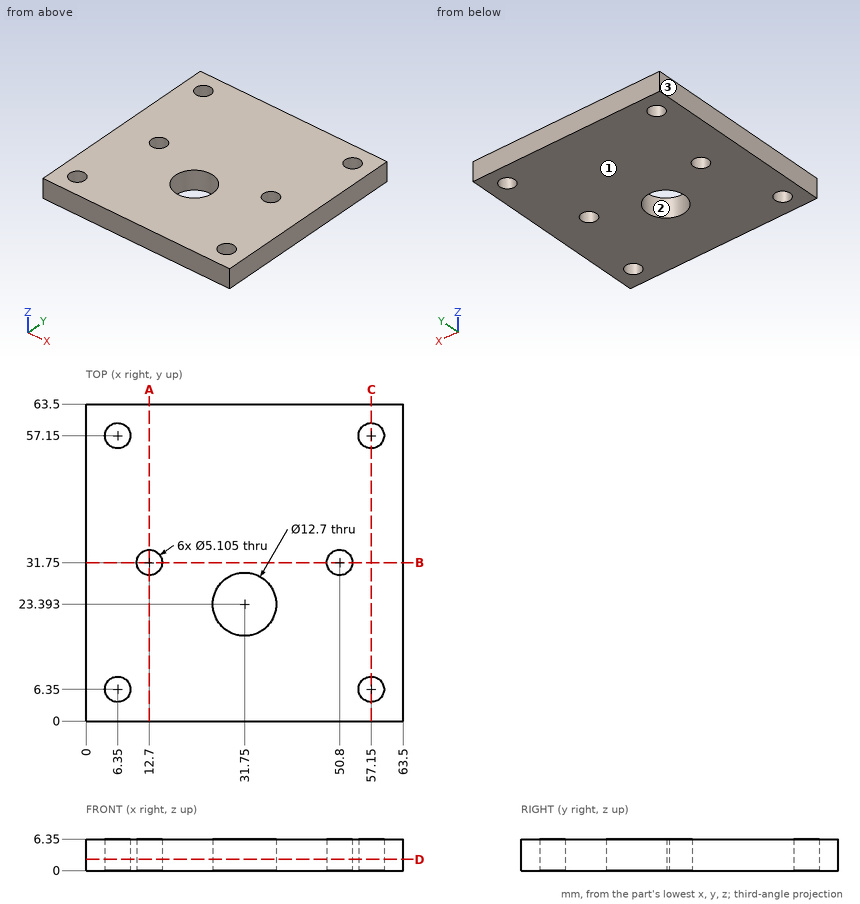
Verification items for this drawing (mm, ordinates from the low corner). Give positions to 0.01 mm unless a question says otherwise; leave off trailing zeros. Write each loop counter-clockwise with the first axis right and the second up, starting at its lowest first coordinate (ties: lowest second). Pieces come first, ordered by that corner, then holes.
1) Cross-section at D-D (z = 2.25). Count the separate pieces of the cut face and the enclosed holes in it, plus the area to 3 significant figures.
Values follow:
separate pieces: 1
enclosed holes: 7
area: 3,780 mm2
2) Cross-section at A-A (x = 12.7). Record the boundary of the cut face in (y, z).
Values follow:
outline: (0, 0) - (29.2, 0) - (29.2, 6.35) - (0, 6.35) - close; (34.3, 0) - (63.5, 0) - (63.5, 6.35) - (34.3, 6.35) - close
3) Release check for a two-part mould opening along X. For the marked faces 1, 2 and 3 record: released by +X, released by -X, zero draft, split by the parting line, or undercut.
Values follow:
face 1: zero draft
face 2: undercut
face 3: released by -X
4) Thickness scan on line 1 (X direction, y = 31.5, z = 2.5); line 2 (Y direction, x = 57.15, z = 3); line 3 (Y direction, x = 59, z = 4.25). Record the ranges inside material, lowest first.
Values follow:
line 1: x = 0 to 10.16, 15.24 to 48.26, 53.34 to 63.5
line 2: y = 0 to 3.8, 8.9 to 54.6, 59.7 to 63.5
line 3: y = 0 to 4.59, 8.11 to 55.39, 58.91 to 63.5
5) Cross-section at B-B (y = 31.75). Record the boundary of the cut face in (x, z).
Values follow:
outline: (0, 0) - (10.15, 0) - (10.15, 6.35) - (0, 6.35) - close; (15.25, 0) - (48.25, 0) - (48.25, 6.35) - (15.25, 6.35) - close; (53.35, 0) - (63.5, 0) - (63.5, 6.35) - (53.35, 6.35) - close
6) Cross-section at C-C (x = 57.15). Record the boundary of the cut face in (y, z).
Values follow:
outline: (0, 0) - (3.8, 0) - (3.8, 6.35) - (0, 6.35) - close; (8.9, 0) - (54.6, 0) - (54.6, 6.35) - (8.9, 6.35) - close; (59.7, 0) - (63.5, 0) - (63.5, 6.35) - (59.7, 6.35) - close
